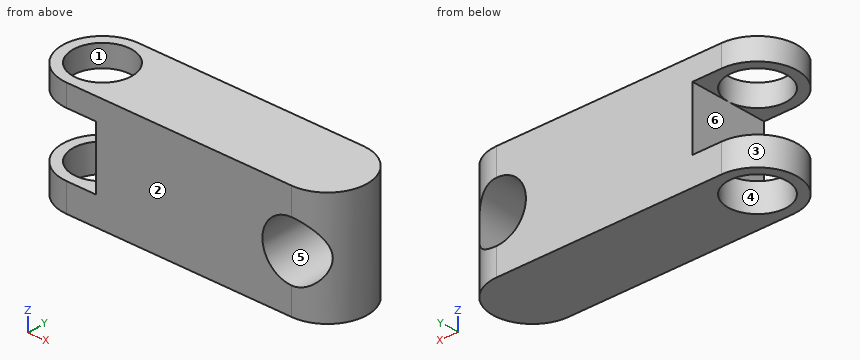
Autodesk Inventor part; units mm, degrees
ref_plane "YZ Plane" through (0, 0, 0) normal (1, 0, 0) x (0, 1, 0)
ref_plane "XZ Plane" through (0, 0, 0) normal (0, 1, 0) x (-1, 0, 0)
ref_plane "XY Plane" through (0, 0, 0) normal (0, 0, 1) x (1, 0, 0)
sketch "Sketch1" plane through (0, 0, 0) normal (0, 0, 1) x (1, 0, 0)
  circle A0 centre (0, 0) radius 6.604
  arc A1 (0, 8.89) -> (0, -8.89) centre (0, 0) ccw
  line L0 (0, 8.89) -> (50.8, 8.89)
  arc A2 (50.8, -8.89) -> (50.8, 8.89) centre (50.8, 0) ccw
  line L1 (0, -8.89) -> (50.8, -8.89)
  dimension "d0" = 13.208
  dimension "d1" = 17.78
  dimension "d2" = 50.8
extrude "Extrusion1" add sketch "Sketch1" along normal blind 25.4
sketch "Sketch2" plane through (0, 0, 0) normal (0, 1, 0) x (-1, 0, 0)
  line L0 (0, 0) -> (0, 25.4)
  line L1 (0, 0) -> (0, 25.4)
  line L2 (8.89, 0) -> (0, 0)
  line L3 (0, 0) -> (0, 12.7)
  line L4 (0, 12.7) -> (0, 25.4)
  line L5 (8.89, 0) -> (8.89, 25.4)
  line L6 (0, 6.35) -> (8.89, 6.35)
  line L7 (8.89, 6.35) -> (8.89, 20.4788)
  line L8 (8.89, 20.4788) -> (0, 20.4788)
  line L9 (0, 20.4788) -> (0, 6.35)
  line L10 (-6.604, 25.4) -> (-6.604, 0)
  line L11 (0, 6.35) -> (-6.604, 6.35)
  line L12 (-6.604, 6.35) -> (-6.604, 20.4788)
  line L13 (-6.604, 20.4788) -> (0, 20.4788)
  line L14 (0, 20.4788) -> (0, 6.35)
extrude "Extrusion2" cut sketch "Sketch2" along normal mid plane 25.4 contours L11 L10 L13 L0 | L0 L8 L5 L6
sketch "Sketch3" plane through (0, 0, 0) normal (0, 1, 0) x (-1, 0, 0)
  line L0 (-50.8, 0) -> (-50.8, 25.4)
  circle A0 centre (-50.8, 12.7) radius 6.604
  point P0 (0, 0)
  dimension "d8" = 13.208
extrude "Extrusion3" cut sketch "Sketch3" along normal mid plane 25.4
properties part number "uperlegV1"
Input: part model. Units: mm. Frame: model coordinates. Face numbers are marked on the shaded views. A direction names the side the tool comes from. Round coordinates to 2 decimals unless told otherwise and drop trailing zeros. Loops run counter-clockwise (first coordinate to the right, second up) from the corner with the lowest first, then second, coordinate; pieces in that order, holes last. Notation, with made-up numbers: (-38, 1.25) -> (6, 1.25) arc R13 ccw to (6, 23.25) -> close; hole circle Ø2 at (-1.5, 27.5). An arc over 180 degrees is marked (long way). Write each question's results on one line, items separated by ' | '.
1. Mould query, pull axis Y, two halves, no side actions, for the marked faces 1, 2, 3 and 4. Classes: +Y half, -Y half, draft (parallel to the pull), parting line (faces both ways), or undercut.
Geometry results:
face 1: undercut | face 2: -Y half | face 3: parting line | face 4: undercut
2. Ray query, line 1 (X direction, y = 0, z = 2.75); line 2 (Z direction, x = 0.5, y = 6.75); line 3 (Y direction, x = 0, z = 24.2). Return the intervals inside material, ascending. Write a range as from..to.
Geometry results:
line 1: -8.89..-6.6, 6.6..59.69 | line 2: 0..6.35, 20.48..25.4 | line 3: -8.89..-6.6, 6.6..8.89
3. Set-up query: the marked faces 5 and 6. Return all of +Z, -Z, +X, -X, +Y, -Y with unobstructed straight access to the full face (end or side cutting, diameter ignored); none if empty.
Geometry results:
face 5: +Y, -Y | face 6: -X, +Y, -Y
4. Section C-C (x = 4). Return loops of the section in (y, z), and give its area (3 significant figures).
Geometry results:
outline: (-8.89, 0) -> (-5.25, 0) -> (-5.25, 6.35) -> (-8.89, 6.35) -> close; (-8.89, 20.48) -> (-5.25, 20.48) -> (-5.25, 25.4) -> (-8.89, 25.4) -> close; (5.25, 0) -> (8.89, 0) -> (8.89, 6.35) -> (5.25, 6.35) -> close; (5.25, 20.48) -> (8.89, 20.48) -> (8.89, 25.4) -> (5.25, 25.4) -> close | area: 81.9 mm2
5. Section A-A (y = -4.25). Return loops of the section in (x, z), and give its area (3 significant figures).
Geometry results:
outline: (-7.81, 0) -> (-5.05, 0) -> (-5.05, 6.35) -> (-7.81, 6.35) -> close; (-7.81, 20.48) -> (-5.05, 20.48) -> (-5.05, 25.4) -> (-7.81, 25.4) -> close; (5.05, 0) -> (58.61, 0) -> (58.61, 25.4) -> (5.05, 25.4) -> (5.05, 20.48) -> (6.6, 20.48) -> (6.6, 6.35) -> (5.05, 6.35) -> close; hole circle Ø13.21 at (50.8, 12.7) | area: 1,230 mm2
6. Section B-B (z = 23). Return loops of the section in (x, y), and give its area (3 significant figures).
Geometry results:
outline: (0, -8.89) -> (50.8, -8.89) arc R8.89 ccw to (50.8, 8.89) -> (0, 8.89) arc R8.89 ccw to start; hole circle Ø13.21 at (0, 0) | area: 1,010 mm2
7. First-contact query: P1, Ø4, axis at y = -3, z = 13, coming from the +X side; P2, Ø3, axis at y = -2, z = 9.5, coming from the +X side; P3, Ø2, axis at y = -1.5, z = 22.5, coming from the -X side; P4, Ø10.5, axis at x = 0, y = 0, coming from the -Z side. Flat tips, straight axial feed; report the tip coordinate or a pass-through.
Geometry results:
P1: x = 59.63 | P2: x = 59.68 | P3: x = -8.88 | P4: through
8. Section D-D (z = 8.25). Return loops of the section in (x, y).
Geometry results:
outline: (6.6, -8.89) -> (45.92, -8.89) -> (45.92, 8.89) -> (6.6, 8.89) -> close; (55.68, -7.43) arc R8.89 ccw to (55.68, 7.43) -> close
